For this review, take the finished solid that the model builds, in its own axes (mm). A direction names the side the tool comes from. Round coordinates to 2 decimals unless told otherwise and drop trailing zeros. Loops run counter-clockwise (first coordinate to the right, second up) from the corner with the lowest first, then second, coordinate; pieces in that order, holes last.
1) Take a section at A-A (x = 47.5). State the section outline as (y, z) points.
2) Mouldability with a two-part tool opening along Z and no side actions: class faces 1 (the flat face through (-16, 20, 28)), 2 (the flat face through (-53, 10, 25.226)), 3 (the flat face through (-6, 10, -25.999)) as pulls with the +Z half, pulls with the -Z half, needs draft (parallel to the pull), parting line crosses it, or undercut.
3) Wall thickness on L1, parallel to X at y = 19.25, z = -12; L2, parallel to Z at x = -51, y = 5.5; L3, parallel to X at y = 11.25, z = 13: over which ranges is each line inside the solid? List them lowest first.
4) Take a section at D-D (x = -12). State the section outline as (y, z) points.
5) Take a section at C-C (y = 16.25). State the section outline as (x, z) points, then the cut area to 3 significant figures.
6) Tool access review of faces 4 (the flat face through (-1, 19, 2)), 5 (the flat face through (-53, 10, -21.647)), 6 (the flat face through (51, 10, 25.226)): name each direction out of +Z, -Z, +X, -X, +Y, -Y from which nothing blocks a thin tool from reaching the whole face with its end or side.
7) Insertion check: pin 1 (5 mm diameter, centred on x = 22, z = -9, fed in from +Y); pin 2 (0.8 mm diameter, centred on y = 19.5, z = 11, fed in from +X); pin 3 (1.7 mm diameter, centred on y = 5, z = 28.5, fed in from -X). Each pin has a flat end and moves straight along its axis. Give the tip position at first contact, or say it passes through.
8) Take a section at B-B (z = 19). State the section outline as (x, y) points, then the cut area to 3 significant figures.
```python
from build123d import *

# Parameters (mm, degrees)
BOSS_EXTRUDE1_DEPTH = 20
SKETCH2_R           = 9.180948857
BOSS_EXTRUDE2_DEPTH = 16.762555
SKETCH3_W           = 74.249943047
SKETCH3_H           = 48.931949377
CUT_EXTRUDE1_DEPTH  = 1


with BuildPart() as part:
    # Sketch1 → Boss-Extrude1 (new body)
    with BuildSketch(Plane(origin=(0, 0, 0), x_dir=(1, 0, 0), z_dir=(0, 1, 0))):
        Polygon((-50.055146164, 21.646889896), (-50.055146164, -25.226179967), (-55.206550944, -25.226179967), (-55.206550944, -30.910542614), (-31.621863062, -30.910542614), (17.979762571, -30.910542614), (59.391812496, -30.910542614), (59.391812496, -25.226179967), (42.62925771, -25.226179967), (42.62925771, 25.999180786), (-46.65640648, 25.999180786), (-56.142161298, 25.999180786), (-56.142161298, 21.646889896), align=None)
    extrude(amount=BOSS_EXTRUDE1_DEPTH)

    # Sketch2 → Boss-Extrude2 (add)
    with BuildSketch(Plane(origin=(42.62925771, 0, 0), x_dir=(0, 0, -1), z_dir=(1, 0, 0))):
        with Locations(Location((15.911282323, 9.888690044, 0), (0, 0, 180))):  # turned: the seam where the file's is
            Circle(SKETCH2_R)
    extrude(amount=BOSS_EXTRUDE2_DEPTH)

    # Sketch3 → Cut-Extrude1 (cut)
    with BuildSketch(Plane(origin=(0, 20, 0), x_dir=(1, 0, 0), z_dir=(0, 1, 0))):
        with Locations((-0.592763324, -2.194150519)):
            Rectangle(SKETCH3_W, SKETCH3_H)
    extrude(amount=-CUT_EXTRUDE1_DEPTH, mode=Mode.SUBTRACT)


solid = part.part
```
Response:
1. outline: (0, 25.23) - (20, 25.23) - (20, 30.91) - (0, 30.91) - close; circle Ø18.36 at (9.89, -15.91)
2. face 1: needs draft
2. face 2: undercut
2. face 3: pulls with the -Z half
3. L1: x = -50.06 to -37.72, 36.53 to 42.63
3. L2: z = -26 to -21.65, 25.23 to 30.91
3. L3: x = -50.06 to 42.63
4. outline: (0, -26) - (20, -26) - (20, -22.27) - (19, -22.27) - (19, 26.66) - (20, 26.66) - (20, 30.91) - (0, 30.91) - close
5. outline: (-56.14, -26) - (42.63, -26) - (42.63, -22.53) - (59.39, -22.53) - (59.39, -9.29) - (42.63, -9.29) - (42.63, 25.23) - (59.39, 25.23) - (59.39, 30.91) - (-55.21, 30.91) - (-55.21, 25.23) - (-50.06, 25.23) - (-50.06, -21.65) - (-56.14, -21.65) - close
5. area: 5,650 mm2
6. face 4: +Y
6. face 5: -X, +Y, -Y
6. face 6: +X, +Y, -Y
7. pin 1: stops at y = 19
7. pin 2: stops at x = 42.63
7. pin 3: stops at x = -55.21
8. outline: (-50.06, 0) - (42.63, 0) - (42.63, 20) - (36.53, 20) - (36.53, 19) - (-37.72, 19) - (-37.72, 20) - (-50.06, 20) - close
8. area: 1,780 mm2
